Work out the finished part from the listing and answer in its coordinate system (mm). A direction names the side the tool comes from. Give positions to 0.01 mm unless a question says otherwise; leave off trailing zeros. Write each loop counter-clockwise with the first axis right and the second up, starting at its lowest first coordinate (ties: lowest second). Pieces come first, ordered by that corner, then holes.
1) Given pin 1 Ø1.5 at (y, z) = (-61.5, 9) entering from +X; pin 2 Ø10 at (y, z) = (18.5, 9.5) entering from -X; pin 3 Ø1.5 at (x, z) = (34, 42.5) entering from -Y; pin 4 Ø1 at (x, y) = (19, -55.5) entering from +Z, each flat-ended and moving along its own axis, determine where each tip first touches the part or whether it passes through.
2) Find section B-B (x = 20.32). Determine the outline of the cut face in (y, z), plus the area to 3 significant figures.
3) Straight lines are drawn through the part: probe 1 along Z at (x, y) = (17.5, 26); probe 2 along Y at (x, z) = (12, 4.5); probe 3 along Y at (x, z) = (33, 37.5). For each, find the intervals that lie inside material, in ascending order.
4) A tool of negligible diameter and unlimited length cuts with its end or side. For faces 4 (the face through (43.68, 18.58, 37.92)), 5 (the face through (25, 50.8, 13)), 6 (the face through (12.257, -37.567, 6.518)), from which of +Z, -Z, +X, -X, +Y, -Y can it reach the whole face along a straight path? Write none if from no direction.
5) Find section A-A (z = 12.7). Determine the outline of the cut face in (x, y), plus the area to 3 significant figures.
6) Find section C-C (y = -36). Determine the outline of the cut face in (x, z), plus the area to 3 significant figures.
7) Find section D-D (z = 37.5). Determine the outline of the cut face in (x, y), plus the area to 3 significant figures.
8) Determine the mould class of faces 1 (the face through (25, 26, 0)), 2 (the face through (50.8, 25, 13)), 3 (the face through (35, 22, 50.8)) for opening direction Z: pulls with the +Z half, pulls with the -Z half, needs draft (parallel to the pull), parting line crosses it, or undercut.
```python
from build123d import *

# Parameters (mm, degrees)
F0_W     = 50.8
F0_H     = 50.8
F1_DEPTH = 25.4
F2_R     = 10.16
F3_DEPTH = 76.2
F4_R     = 9.221504
F5_DEPTH = 25.4


with BuildPart() as f1:
    # F0 (on Top) → F1 (new body)
    with BuildSketch(Plane.XY):
        with Locations((25.4, 25.4)):
            Rectangle(F0_W, F0_H)
    extrude(amount=F1_DEPTH)

    # F2 (on face) → F3 (join)
    with BuildSketch(Plane.XZ):
        with Locations((20.32, 12.7)):
            Circle(F2_R)
    extrude(amount=F3_DEPTH)

    # F4 (on face) → F5 (join)
    with BuildSketch(Plane.XY.offset(25.4)):
        with Locations((35.16157, 22.115249)):
            Circle(F4_R)
    extrude(amount=F5_DEPTH)


solid = f1.part
```
Results:
1. pin 1: stops at x = 30.04
1. pin 2: stops at x = 0
1. pin 3: stops at y = 12.9
1. pin 4: stops at z = 22.83
2. outline: (-76.2, 2.54) - (0, 2.54) - (0, 0) - (50.8, 0) - (50.8, 25.4) - (0, 25.4) - (0, 22.86) - (-76.2, 22.86) - close
2. area: 2,840 mm2
3. probe 1: z = 0 to 25.4
3. probe 2: y = 0 to 50.8
3. probe 3: y = 13.15 to 31.08
4. face 4: +Z
4. face 5: +Z, -Z, +X, -X, +Y
4. face 6: -Y
5. outline: (0, 0) - (10.16, 0) - (10.16, -76.2) - (30.48, -76.2) - (30.48, 0) - (50.8, 0) - (50.8, 50.8) - (0, 50.8) - close
5. area: 4,130 mm2
6. outline: circle Ø20.32 at (20.32, 12.7)
6. area: 324 mm2
7. outline: circle Ø18.44 at (35.16, 22.12)
7. area: 267 mm2
8. face 1: pulls with the -Z half
8. face 2: needs draft
8. face 3: pulls with the +Z half
